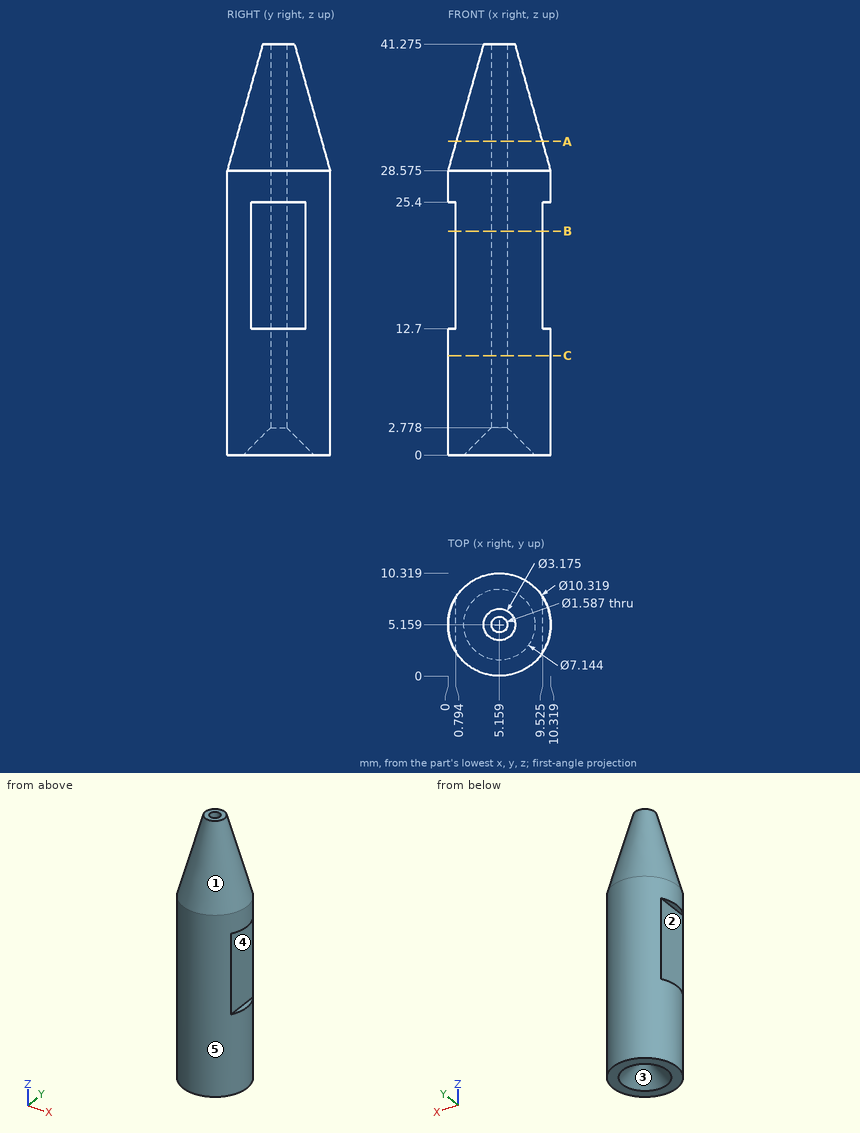
Here's the drawing with two shaded views (mm, measured from the low corner). I have some questions. A direction names the side the tool comes from. Round coordinates to 2 decimals unless told otherwise and drop trailing zeros. Loops run counter-clockwise (first coordinate to the right, second up) from the corner with the lowest first, then second, coordinate; pieces in that order, holes last. Notation, with made-up numbers: M -2.5,-17 L 33.5,-17 A14 ccw 33.5,0 Z; hole C 76.25,-33 d1. An arc over 180 degrees is marked long. Put each result on its own line as item: value.
Q1. For pin 1 (4.5 mm diameter, centred on y = 4.5, z = 18, fed in from +X) (1 decimal); pin 2 (3 mm diameter, centred on y = 5.5, z = 25.5, fed in from -X); pin 3 (1.5 mm diameter, centred on x = 7.5, z = 17, fed in from -Y); pin 4 (1.5 mm diameter, centred on y = 4, z = 21.5, fed in from -X), each with a flat end and sliding along its axis, tell me the tip position at first contact or that it passes through.
Check result:
pin 1: x = 9.5
pin 2: x = 0
pin 3: y = 0.25
pin 4: x = 0.79
Q2. Imagine slicing it at C-C (z = 10). Write out the boundary of the cut face in (x, y).
Check result:
outline: C 5.16,5.16 d10.32; hole C 5.16,5.16 d1.59
Q3. I need wall thicknesses on probe 1 along X at (y, z) = (5.75, 29) (1 decimal); probe 2 along Y at (x, z) = (5.25, 24); probe 3 along X at (y, z) = (4.75, 23.5) (1 decimal). Which ranges of each line are inside material? Lowest first, please.
Check result:
probe 1: 0.2 to 4.6, 5.7 to 10.2
probe 2: 0 to 4.37, 5.95 to 10.32
probe 3: 0.8 to 4.5, 5.8 to 9.5
Q4. Imagine slicing it at A-A (z = 31.5). Write out the boundary of the cut face in (x, y), then the cut area to 3 significant figures.
Check result:
outline: C 5.16,5.16 d8.67; hole C 5.16,5.16 d1.59
area: 57.1 mm2
Q5. On a 3-axis mill with a long thin cutter (end or side, diameter ignored), from which of +Z, -Z, +X, -X, +Y, -Y can I reach the whole of each face in a straight line? I mean the marked faces 4 and 5. Say none if no direction works.
Check result:
face 4: +X, +Y, -Y
face 5: +Z, -Z
Q6. Thinking about a two-plate mould opening in Z: for the marked faces 1, 2 and 3, which applies, released by +Z, released by -Z, zero draft, split by the parting line, or undercut?
Check result:
face 1: released by +Z
face 2: undercut
face 3: released by -Z
Q7. Imagine slicing it at B-B (z = 22.5). Write out the boundary of the cut face in (x, y) (1 decimal).
Check result:
outline: M 0.8,2.4 A5.2 ccw 9.5,2.4 L 9.5,7.9 A5.2 ccw 0.8,7.9 Z; hole C 5.2,5.2 d1.6
